from build123d import *

# Parameters (mm, degrees)
F0_W      = 48
F0_H      = 165
F1_DEPTH  = 50
F2_W      = 115
F2_H      = 28
F3_DEPTH  = 48
F4_R      = 9.525
F5_DEPTH  = 25
F6_SIZE   = 7
F7_SIZE   = 6
F9_DEPTH  = 165
F10_R     = 2.25
F11_DEPTH = 25
F10_R_2   = 4
F12_DEPTH = 5
F14_DEPTH = 48
F15_R     = 3
F16_DEPTH = 14


with BuildPart() as f1:
    # F0 (on Top) → F1 (new body)
    with BuildSketch(Plane.XY):
        Rectangle(F0_W, F0_H)
    extrude(amount=F1_DEPTH)

    # F2 (on face) → F3 (cut)
    with BuildSketch(Plane.YZ.offset(24)):
        with Locations((0, 36)):
            Rectangle(F2_W, F2_H)
    extrude(amount=-F3_DEPTH, mode=Mode.SUBTRACT)

    # F4 (on face) → F5 (cut)
    with BuildSketch(Plane.XZ.offset(82.5)):
        with Locations((0, 37.5)):
            Circle(F4_R)
    extrude(amount=-F5_DEPTH, mode=Mode.SUBTRACT)

    # F6
    f6_edges = [f1.edges().sort_by_distance(p)[0] for p in [
        (-24, -70, 50),
        (24, -70, 50),
    ]]
    chamfer(f6_edges, length=F6_SIZE)

    # F7
    f7_edges = [f1.edges().sort_by_distance(p)[0] for p in [
        (0, 82.5, 50),
    ]]
    chamfer(f7_edges, length=F7_SIZE)

    # F8 (on face) → F9 (cut)
    with BuildSketch(Plane(origin=(0, 82.5, 0), x_dir=(-1, 0, 0), z_dir=(0, 1, 0))):
        Polygon((-11.6835255176, 0), (0, 0), (10.3664744824, 0), (10.3664744824, 13), (5.3664744824, 13), (5.3664744824, 22), (-6.6835255176, 22), (-6.6835255176, 13), (-11.6835255176, 13), align=None)
    extrude(amount=-F9_DEPTH, mode=Mode.SUBTRACT)

    # F10 (on face) → F11 (cut)
    with BuildSketch(Plane(origin=(0, 82.5, 0), x_dir=(-1, 0, 0), z_dir=(0, 1, 0))):
        with Locations((16, 34)):
            Circle(F10_R)
        with Locations((-16, 34)):
            Circle(F10_R)
    extrude(amount=-F11_DEPTH, mode=Mode.SUBTRACT)

    # F10 (on face) → F12 (cut)
    with BuildSketch(Plane(origin=(0, 82.5, 0), x_dir=(-1, 0, 0), z_dir=(0, 1, 0))):
        with Locations((-16, 34)):
            Circle(F10_R_2)
        with Locations((-16, 34)):
            Circle(F10_R, mode=Mode.SUBTRACT)
        with Locations((16, 34)):
            Circle(F10_R_2)
        with Locations((16, 34)):
            Circle(F10_R, mode=Mode.SUBTRACT)
    extrude(amount=-F12_DEPTH, mode=Mode.SUBTRACT)

    # F13 (on face) → F14 (cut)
    with BuildSketch(Plane(origin=(-24, 0, 0), x_dir=(0, -1, 0), z_dir=(-1, 0, 0))):
        with BuildLine():
            Line((82.5, 9), (21.3676690006, 3.9978104641))
            ThreePointArc((21.3676690006, 3.9978104641), (18.6251674833, 2.781247562), (17.5, 0))
            Line((17.5, 0), (82.5, 0))
            Line((82.5, 0), (82.5, 9))
        make_face()
    extrude(amount=-F14_DEPTH, mode=Mode.SUBTRACT)

    # F15 (on face) → F16 (cut)
    with BuildSketch(Plane(origin=(0, 0, 0), x_dir=(1, 0, 0), z_dir=(0, 0, -1))):
        with Locations((-17.1832372412, -0.5)):
            Circle(F15_R)
        with Locations((-17.1832372412, -56.5)):
            Circle(F15_R)
        with Locations((17.8167627588, -56.5)):
            Circle(F15_R)
        with Locations((17.8167627588, -0.5)):
            Circle(F15_R)
    extrude(amount=-F16_DEPTH, mode=Mode.SUBTRACT)


solid = f1.part
CAD build for the part. Positions are in the model's coordinates, mm. A direction names the side the tool comes from. Round coordinates to 2 decimals unless told otherwise and drop trailing zeros. Loops run counter-clockwise (first coordinate to the right, second up) from the corner with the lowest first, then second, coordinate; pieces in that order, holes last.
(1) Wall check: line 1 along X through (y, z) = (56.5, 5.5); line 2 along Y through (x, z) = (13, 25); line 3 along X through (y, z) = (43.5, 18.5). Give the ranges that are in metal, low to high.
(2) Drop flat-ended pins along their axis: pin 1 (9.5 mm diameter, centred on x = 17.82, y = 0.5, fed in from +Z); pin 2 (3 mm diameter, centred on x = -16, y = 1, fed in from -Z); pin 3 (6.5 mm diameter, centred on x = 16, z = 34, fed in from +Y). Give the stop position or say it passes through.
(3) Which spindle directions (+Z, -Z, +X, -X, +Y, -Y) get a long thin tool onto all of the face, cutting with end or side? Do faces 5 (the flat face through (1, -70, 22)), 6 (the flat face through (0, 57.5, 36)), 7 (the flat face through (-18, 77.5, 32)). Say none if no direction does.
(4) Cut at D-D (z = 34). Give the cut face in (x, y).
(5) Cut at C-C (z = 7.5). Give the cut face in (x, y).
(6) Cut at B-B (y = -6.5). Give the cut face in (x, z), plus the area to 3 significant figures.
(7) Two-plate mould, pull along Z, no slides. Class faces 1 (the cylindrical face through (-20.18, 0.37, 6.9)), 2 (the flat face through (-15, -1, 22)), 3 (the cylindrical face through (14.79, 67.64, 35.897)), 4 (the cylindrical face through (-17.21, 67.64, 35.897)): +Z half, -Z half, draft (parallel to the pull), parting line (faces both ways), or undercut.
(8) Cut at A-A (x = 0). Give the cut face in (y, z) (3 decimals), plus the area to 3 significant figures.
Findings below:
1. line 1: x = -24 to -20.18, -14.18 to -10.37, 11.68 to 14.82, 20.82 to 24
1. line 2: y = -82.5 to -57.5, 57.5 to 82.5
1. line 3: x = -24 to -5.37, 6.68 to 24
2. pin 1: stops at z = 22
2. pin 2: stops at z = 14
2. pin 3: stops at y = 77.5
3. face 5: -Z, +Y, -Y
3. face 6: +Z, +X, -X
3. face 7: +Y
4. outline: (-24, -82.5) - (-8.86, -82.5) - (-8.86, -57.5) - (-24, -57.5) - close; (-24, 57.5) - (-18.25, 57.5) - (-18.25, 77.5) - (-20, 77.5) - (-20, 82.5) - (-24, 82.5) - close; (-13.75, 57.5) - (13.75, 57.5) - (13.75, 77.5) - (12, 77.5) - (12, 82.5) - (-12, 82.5) - (-12, 77.5) - (-13.75, 77.5) - close; (8.86, -82.5) - (24, -82.5) - (24, -57.5) - (8.86, -57.5) - close; (18.25, 57.5) - (24, 57.5) - (24, 82.5) - (20, 82.5) - (20, 77.5) - (18.25, 77.5) - close
5. outline: (-24, -64.17) - (-10.37, -64.17) - (-10.37, 82.5) - (-24, 82.5) - close; (11.68, -64.17) - (24, -64.17) - (24, 82.5) - (11.68, 82.5) - close; hole circle Ø6 at (-17.18, 0.5); hole circle Ø6 at (-17.18, 56.5); hole circle Ø6 at (17.82, 0.5); hole circle Ø6 at (17.82, 56.5)
6. outline: (-24, 0) - (-10.37, 0) - (-10.37, 13) - (-5.37, 13) - (-5.37, 22) - (-24, 22) - close; (6.68, 13) - (11.68, 13) - (11.68, 0) - (24, 0) - (24, 22) - (6.68, 22) - close
6. area: 661 mm2
7. face 1: draft
7. face 2: +Z half
7. face 3: undercut
7. face 4: undercut
8. outline: (-82.5, 22) - (-57.5, 22) - (-57.5, 27.975) - (-82.5, 27.975) - close; (-82.5, 47.025) - (-57.5, 47.025) - (-57.5, 50) - (-82.5, 50) - close; (57.5, 22) - (82.5, 22) - (82.5, 44) - (76.5, 50) - (57.5, 50) - close
8. area: 906 mm2
